Geometry: see drawing. Coordinates: mm, zero at the bounding-box minimum. Give positions to 0.01 mm unless a question says otherwise; leave off trailing zeros. Write each loop counter-clockwise with the first axis right and the second up, starting at its lowest first coordinate (ties: lowest second). Pieces come first, ordered by that corner, then holes. Notation, with made-up numbers: M 24,49 L 60,49 A13 cw 60,73 Z; hole C -27.75,55.25 d2. An arc over 180 degrees is marked long. Use one line per item in the form item = value. Start each with the question number.
Item 1: Section query B-B on y = 21. Return loops of the section in (x, z).
Item 2: Contact query for a flat-ended pin moving along its axis: P1, Ø2.5, axis at x = 23.5, y = 23.5, coming from the +Z side. Output: stop coordinate, or through.
Item 3: Material intervals for line 1 along Y through (x, z) = (23.5, 0.4); line 2 along Y through (x, z) = (13.5, 1); line 3 along Y through (x, z) = (2.5, 1.35), sorted ascending. Write a range as from..to.
Item 4: Section query C-C on z = 0.5. Return loops of the section in (x, y), then the cut area to 3 significant figures.
Item 5: Section query D-D on x = 23.5. Return loops of the section in (y, z).
Item 6: Section query A-A on x = 17.5. Return loops of the section in (y, z).
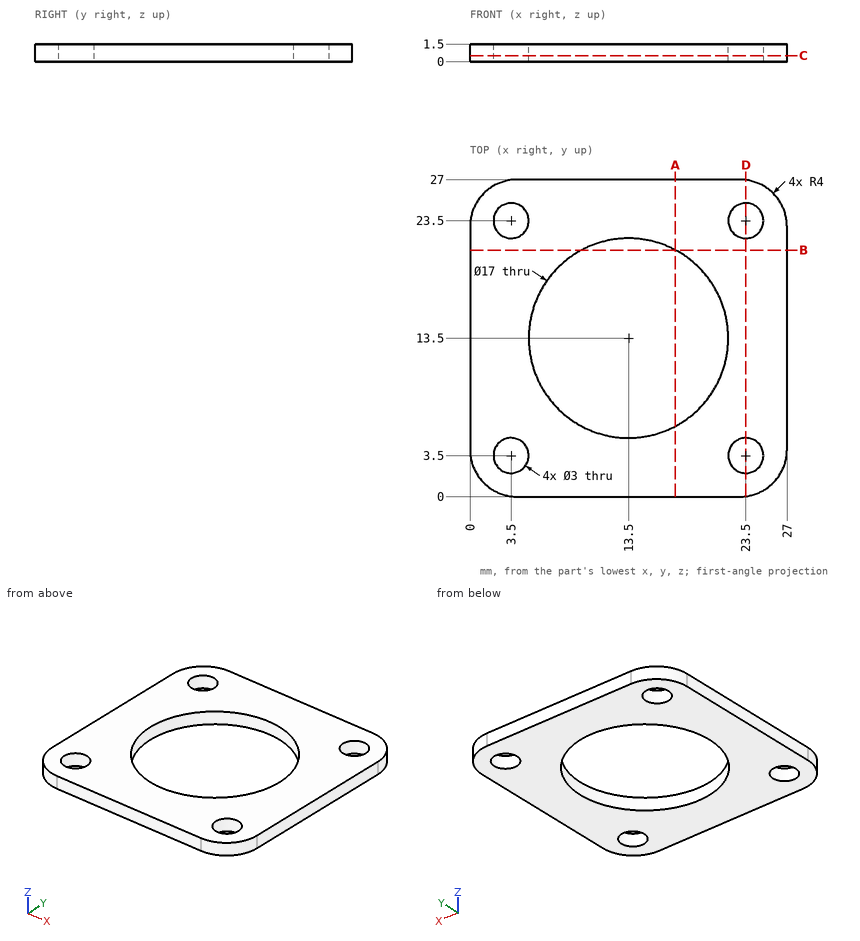
Answer sheet:
q1.outline = M 0,0 L 9.5,0 L 9.5,1.5 L 0,1.5 Z; M 17.5,0 L 27,0 L 27,1.5 L 17.5,1.5 Z
q2.P1 = through
q3.line_1 = 0.03..2, 5..22, 25..26.97
q3.line_2 = 0..5, 22..27
q3.line_3 = 0.29..2.38, 4.62..22.38, 24.62..26.71
q4.outline = M 0,4 A4 ccw 4,0 L 23,0 A4 ccw 27,4 L 27,23 A4 ccw 23,27 L 4,27 A4 ccw 0,23 Z; hole C 3.5,3.5 d3; hole C 3.5,23.5 d3; hole C 13.5,13.5 d17; hole C 23.5,3.5 d3; hole C 23.5,23.5 d3
q4.area = 460 mm2
q5.outline = M 0.03,0 L 2,0 L 2,1.5 L 0.03,1.5 Z; M 5,0 L 22,0 L 22,1.5 L 5,1.5 Z; M 25,0 L 26.97,0 L 26.97,1.5 L 25,1.5 Z
q6.outline = M 0,0 L 6,0 L 6,1.5 L 0,1.5 Z; M 21,0 L 27,0 L 27,1.5 L 21,1.5 Z
